```python
from build123d import *

# Parameters (mm, degrees)
SKETCH8_R           = 85
BOSS_EXTRUDE5_DEPTH = 20
DOME4_FACE_RADIUS   = 85
DOME4_HEIGHT        = 20
HOLE5_OUTLINE_R     = 80
HOLE5_DEPTH         = 16


# Read off the part's stored shape, not the designer's step: Hole5
with BuildPart() as part:
    # Sketch8 → Boss-Extrude5 (new body)
    with BuildSketch(Plane.XY):
        Circle(SKETCH8_R)
    extrude(amount=BOSS_EXTRUDE5_DEPTH)

    # Dome4: a dome of height H over a round flat face of radius A is a cap of a sphere of radius (A * A + H * H) / (2 * H)
    dome4_r = (DOME4_FACE_RADIUS * DOME4_FACE_RADIUS + DOME4_HEIGHT * DOME4_HEIGHT) / (2 * DOME4_HEIGHT)
    dome4_base = Plane((0, 0, 20), z_dir=(0, 0, 1))
    with Locations(dome4_base.offset(DOME4_HEIGHT - dome4_r)):
        dome4_ball = Sphere(dome4_r, mode=Mode.PRIVATE)
    add(split(dome4_ball, bisect_by=dome4_base, keep=Keep.TOP, mode=Mode.PRIVATE))

    # Hole5 outline → Hole5 (cut)
    with BuildSketch(Plane.XY):
        with Locations((-0.204435363, 1.845559102)):
            Circle(HOLE5_OUTLINE_R)
    extrude(amount=HOLE5_DEPTH, mode=Mode.SUBTRACT)


solid = part.part
```
Build history of the part. All positions in model axes, mm. Give positions to 0.01 mm unless a question says otherwise; leave off trailing zeros. Loops run counter-clockwise (first coordinate to the right, second up) from the corner with the lowest first, then second, coordinate; pieces in that order, holes last.
Item 1: Drill centre lines: line 1 (Y direction, x = -67, z = 12); line 2 (Y direction, x = -12, z = 10.5); line 3 (X direction, y = 6, z = 15). Where is each one in solid material? Low to high.
Answers follow:
line 1: y = -52.31 to -42.18, 45.87 to 52.31
line 2: y = -84.15 to -77.28, 80.97 to 84.15
line 3: x = -84.79 to -80.1, 79.69 to 84.79
Item 2: Slice it at A-A, the plane y = -13.5. List the corners of the cut face in (x, z) (3 decimals).
Answers follow:
outline: (-83.921, 0) - (-78.719, 0) - (-78.719, 16) - (78.31, 16) - (78.31, 0) - (83.921, 0) - (83.921, 20) arc R190.146 ccw to (-83.921, 20) - close
Item 3: Slice it at B-B, the plane x = 0. List the corners of the cut face in (y, z) (3 decimals).
Answers follow:
outline: (-85, 0) - (-78.154, 0) - (-78.154, 16) - (81.845, 16) - (81.845, 0) - (85, 0) - (85, 20) arc R190.625 ccw to (-85, 20) - close
Item 4: Pull direction Y, two halves, no side cores. Call faces 1 (the face through (76.1, 25.88, 7.89)), 2 (the face through (-67.453, -51.721, 9.86)), 3 (the face through (25, -75, 0)): released by +Y, released by -Y, zero draft, split by the parting line, or undercut.
Answers follow:
face 1: undercut
face 2: split by the parting line
face 3: zero draft
Item 5: Slice it at D-D, the plane z = 10.5. List the corners of the cut face in (x, y).
Answers follow:
outline: circle Ø170 at (0, 0); hole circle Ø160 at (-0.2, 1.85)
Item 6: Flat gauge pins, fed straight in: pin 1 (3 mm diameter, centred on x = -35, y = 12, fed in from +Z); pin 2 (5 mm diameter, centred on x = 6.5, y = -33, fed in from +Z); pin 3 (12 mm diameter, centred on x = -13, z = 18.5, fed in from -Y). Where does each tip first touch, or does it go through?
Answers follow:
pin 1: stops at z = 36.67
pin 2: stops at z = 37.44
pin 3: stops at y = -84.71
